Study the drawing (mm; zero at the part's minimum x, y, z) and answer. Give positions to 0.01 mm unless a question says otherwise; leave off trailing zeros. Loops run counter-clockwise (first coordinate to the right, second up) from the corner with the lowest first, then second, coordinate; pieces in that order, holes last. Notation, with made-up numbers: M 63,58 L 120,58 A7 cw 120,66 Z; hole C 31,-32.75 d4. An arc over 180 degrees is marked long. Return JSON: item names as keys, results as strings.
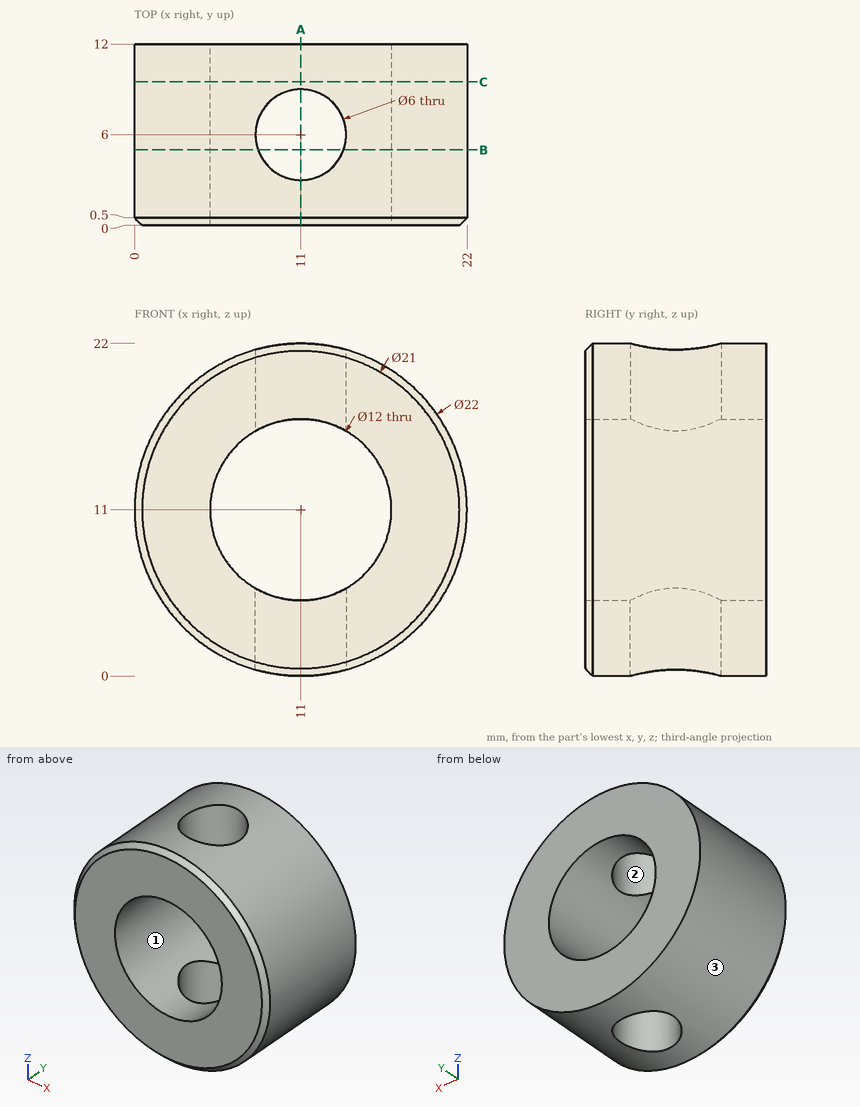
(1) Straight lines are drawn through the part: line 1 along Y through (x, z) = (11, 1.7); line 2 along Z through (x, y) = (15, 8.75); line 3 along Z through (x, y) = (9.5, 2.5). For each, find the intervals that lie inside material, in ascending order.
Values follow:
{"line 1": "0 to 3, 9 to 12", "line 2": "0.75 to 6.53, 15.47 to 21.25", "line 3": "0.1 to 5.19, 16.81 to 21.9"}
(2) Given pin 1 (2 mm diameter, centred on y = 4.5, z = 5.5, fed in from +X); pin 2 (4 mm diameter, centred on x = 16.5, y = 10, fed in from +Z); pin 3 (1.5 mm diameter, centred on y = 7, z = 3.5, fed in from -X); pin 4 (5 mm diameter, centred on x = 11, y = 6, fed in from -Z), each flat-ended and moving along its own axis, determine where each tip first touches the part or whether it passes through.
Values follow:
{"pin 1": "x = 21.04", "pin 2": "z = 21.43", "pin 3": "x = 2.31", "pin 4": "through"}
(3) Determine the mould class of the marked faces 1, 2 and 3 for opening direction Z: released by +Z, released by -Z, zero draft, split by the parting line, or undercut.
Values follow:
{"face 1": "undercut", "face 2": "zero draft", "face 3": "split by the parting line"}
(4) The part is cut by section B-B (y = 5). Determine the outline of the cut face in (x, z), and give its area (3 significant figures).
Values follow:
{"outline": "M 8.17,0.37 L 8.17,5.71 A6 cw 8.17,16.29 L 8.17,21.63 A11 ccw Z; M 13.83,0.37 A11 ccw 13.83,21.63 L 13.83,16.29 A6 cw 13.83,5.71 Z", "area": "209 mm²"}
(5) The part is cut by section A-A (x = 11). Determine the outline of the cut face in (y, z), and give its area (4 significant figures).
Values follow:
{"outline": "M 0,0.5 L 0.5,0 L 3,0 L 3,5 L 0,5 Z; M 0,17 L 3,17 L 3,22 L 0.5,22 L 0,21.5 Z; M 9,0 L 12,0 L 12,5 L 9,5 Z; M 9,17 L 12,17 L 12,22 L 9,22 Z", "area": "59.75 mm²"}
(6) The part is cut by section C-C (y = 9.5). Determine the outline of the cut face in (x, z), and give its area (3 significant figures).
Values follow:
{"outline": "C 11,11 d22; hole C 11,11 d12", "area": "267 mm²"}
